Autodesk Fusion 360 part; units mm, degrees
sketch "Sketch1" plane through (0, 0, 0) normal (0, 0, 1) x (1, 0, 0)
  line L0 (-19.05, -19.05) -> (19.05, -19.05)
  line L1 (19.05, -19.05) -> (19.05, 19.05)
  line L2 (19.05, 19.05) -> (-19.05, 19.05)
  line L3 (-19.05, 19.05) -> (-19.05, -19.05)
  line L4 (0, 1.75) -> (0, 22.5)
  line L5 (1.75, 0) -> (22.5, 0)
  dimension "d1" = 38.1
  dimension "d2" = 38.1
extrude "Extrude1" add sketch "Sketch1" along normal blind 38.1
sketch "Sketch2" plane through (0, 0, 38.1) normal (0, 0, 1) x (-1, 0, 0)
  line L0 (19.05, -19.05) -> (19.05, 19.05)
  line L1 (19.05, 19.05) -> (-19.05, 19.05)
  line L2 (-19.05, 19.05) -> (-19.05, -19.05)
  line L3 (-19.05, -19.05) -> (19.05, -19.05)
  circle A0 centre (0, 0) radius 13.97
  dimension "d5" = 27.94
extrude "Extrude2" cut sketch "Sketch2" against normal blind 25.4 contours A0
sketch "Sketch3" plane through (0, 0, 12.7) normal (0, 0, 1) x (-1, 0, 0)
  circle A0 centre (0, 0) radius 13.97
  circle A1 centre (0, 0) radius 16.51
  dimension "d8" = 2.54
extrude "Extrude3" cut sketch "Sketch3" along normal blind 10.16 contours A0 | A1
chamfer "Chamfer1" distance 2.54 angle 45 1 edges at (13.0246, -5.0518, 22.86)
chamfer "Chamfer2" distance 2.54 angle 45 1 edges at (13.0246, -5.0518, 38.1)
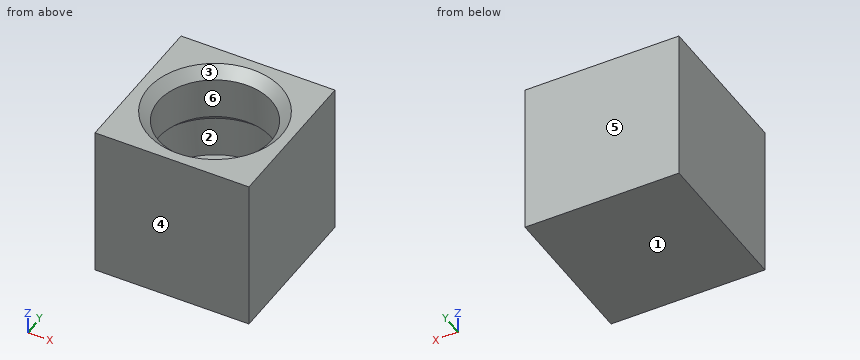
For this review, take the finished solid that the model builds, in its own axes (mm). Face numbers are marked on the shaded views. A direction names the side the tool comes from. Give positions to 0.01 mm unless a question says otherwise; leave off trailing zeros. Order: outer loops, then holes, each group sorted by start corner. A loop starts at its lowest first (then second) coordinate and runs counter-clockwise, first axis right, second up.
1) Take a section at B-B (z = 35). Give the boundary of the cut face in (x, y), then the cut area to 3 significant figures.
2) Wall thickness on line 1 (X direction, y = 0, z = 33); line 2 (X direction, y = 0, z = 19.5): over which ranges is each line inside the solid? List them lowest first.
3) Insertion check: pin 1 (12 mm diameter, centred on x = -11, y = -0.5, fed in from -Z). The pin has a flat end and moves straight along its axis. Give the tip position at first contact, or say it passes through.
4) For the marked faces 5 and 6, list the 3-axis set-ups (+Z, -Z, +X, -X, +Y, -Y) from which the entire face can be reached by the end or side of a thin tool; tool diameter is ignored.
5) The part is to be moulded in two halves that separate along Y. For the marked faces 1, 2, 3 and 4, say which applies: released by +Y, released by -Y, zero draft, split by the parting line, or undercut.
6) Take a section at D-D (z = 20). Give the boundary of the cut face in (x, y), then the cut area to 3 significant figures.
Derived:
1. outline: (-19.05, -19.05) - (19.05, -19.05) - (19.05, 19.05) - (-19.05, 19.05) - close; hole circle Ø27.94 at (0, 0)
1. area: 838 mm2
2. line 1: x = -19.05 to -13.97, 13.97 to 19.05
2. line 2: x = -19.05 to -16.51, 16.51 to 19.05
3. pin 1: stops at z = 0
4. face 5: +Z, -Z, +X, -X, +Y
4. face 6: +Z
5. face 1: zero draft
5. face 2: undercut
5. face 3: undercut
5. face 4: released by -Y
6. outline: (-19.05, -19.05) - (19.05, -19.05) - (19.05, 19.05) - (-19.05, 19.05) - close; hole circle Ø33.02 at (0, 0)
6. area: 595 mm2
